Verification items for the finished model (mm, model axes). A direction names the side the tool comes from. Coordinates: 2 decimals unless noted, no trailing zeros. Order: outer loops, then holes, each group sorted by start corner. A loop starts at its lowest first (then second) coordinate and runs counter-clockwise, first axis right, second up. Notation, with made-up numbers: (71, 3) -> (129, 3) arc R23 ccw to (129, 14) -> close; hole circle Ø7 at (-6.5, 73). An arc over 180 degrees is marked (long way). Write item = value, one per line. Start each with the question number.
Autodesk Inventor part; units mm, degrees
ref_plane "YZ Plane" through (0, 0, 0) normal (1, 0, 0) x (0, 1, 0)
ref_plane "XZ Plane" through (0, 0, 0) normal (0, 1, 0) x (-1, 0, 0)
ref_plane "XY Plane" through (0, 0, 0) normal (0, 0, 1) x (1, 0, 0)
sketch "Эскиз1" plane through (0, 0, 0) normal (0, 1, 0) x (-1, 0, 0)
  circle A0 centre (0, 0) radius 40
  dimension "d0" = 80
extrude "Выдавливание1" add sketch "Эскиз1" along normal blind 90
sketch "Эскиз2" plane through (0, 0, 0) normal (0, 0, 1) x (1, 0, 0)
  line L0 (0, 70) -> (-20, 70)
  line L1 (-20, 70) -> (-20, 90)
  line L2 (0, 70) -> (20, 70)
  line L3 (20, 70) -> (20, 90)
  line L4 (20, 0) -> (20, 20)
  line L5 (20, 20) -> (-40, 70)
  line L6 (-40, 70) -> (-40, 0)
  line L7 (20, 0) -> (-40, 0)
  line L8 (-40, 0) -> (20, 0)
  line L9 (-20, 90) -> (20, 90)
  point P0 (0, 0)
extrude "Выдавливание2" cut sketch "Эскиз2" against normal mid plane 1000
properties part number "Деталь1вар2"
Item 1: Gauge pin test, flat ends, axial feed: P1, Ø12, axis at x = 11.5, y = 75.5, coming from the +Z side; P2, Ø22, axis at y = 5, z = 12, coming from the -X side; P3, Ø3, axis at y = 52, z = 15, coming from the -X side. Record the tip position at first contact, or that the pin passes through.
Item 2: Tool access check on faces 4 (the flat face through (-28, 90, 0)), 5 (the flat face through (20, 10, 0)), 6 (the flat face through (20, 80, 0)). Record the directions out of +Z, -Z, +X, -X, +Y, -Y that give a thin tool (end or side, any length) a straight path to the whole face; none if there is none.
Item 3: Section check B-B (z = 0). Record the boundary of the cut face in (x, y), then the cut area to 3 significant figures.
Item 4: Section check D-D (z = 18). Record the boundary of the cut face in (x, y), then the cut area to 3 significant figures.
Item 5: Thickness scan on line 1 (X direction, y = 79.5, z = -2.5); line 2 (X direction, y = 86.5, z = 28.5); line 3 (X direction, y = 19.5, z = -7.5). Record the ranges inside material, lowest first.
Item 6: Mould release check, pull along X, two halves, no side actions. Record for faces 1 (the flat face through (28, 90, 0)), 2 (the cylindrical face through (39.96, 54.37, -1.76)), 3 (the flat face through (-20, 80, 0)): pulls with the +X half, pulls with the -X half, needs draft (parallel to the pull), parting line crosses it, or undercut.
Item 7: Section check C-C (x = -21.5). Record the boundary of the cut face in (y, z).
Item 8: Section check A-A (y = 78). Record the boundary of the cut face in (x, z), then the cut area to 3 significant figures.
Filled sheet:
q1.P1 = 38.95
q1.P2 = 20
q1.P3 = -20.2
q2.face_4 = +Z, -Z, +X, -X, +Y
q2.face_5 = +Z, -Z, -X, -Y
q2.face_6 = +Z, -Z, +Y
q3.outline = (-40, 70) -> (20, 20) -> (20, 0) -> (40, 0) -> (40, 90) -> (20, 90) -> (20, 70) -> (-20, 70) -> (-20, 90) -> (-40, 90) -> close
q3.area = 3,700 mm^2
q4.outline = (-35.72, 66.43) -> (20, 20) -> (20, 0) -> (35.72, 0) -> (35.72, 90) -> (20, 90) -> (20, 70) -> (-20, 70) -> (-20, 90) -> (-35.72, 90) -> close
q4.area = 3,220 mm^2
q5.line_1 = -39.92 to -20, 20 to 39.92
q5.line_2 = -28.07 to -20, 20 to 28.07
q5.line_3 = 20 to 39.29
q6.face_1 = needs draft
q6.face_2 = parting line crosses it
q6.face_3 = undercut
q7.outline = (54.58, -33.73) -> (90, -33.73) -> (90, 33.73) -> (54.58, 33.73) -> close
q8.outline = (-20, -34.64) -> (-20, 34.64) arc R40 ccw to start; (20, -34.64) arc R40 ccw to (20, 34.64) -> close
q8.area = 1,970 mm^2
